Autodesk Inventor part; units mm, degrees
ref_plane "YZ Plane" through (0, 0, 0) normal (1, 0, 0) x (0, 1, 0)
ref_plane "XZ Plane" through (0, 0, 0) normal (0, 1, 0) x (-1, 0, 0)
ref_plane "XY Plane" through (0, 0, 0) normal (0, 0, 1) x (1, 0, 0)
sketch "Sketch1" plane through (0, 0, 0) normal (0, 0, 1) x (1, 0, 0)
  line L0 (0, 0) -> (50.8, 0)
  line L1 (50.8, 0) -> (50.8, 25.4)
  line L2 (50.8, 25.4) -> (0, 25.4)
  line L3 (0, 25.4) -> (0, 0)
  line L4 (3.175, 3.175) -> (47.625, 3.175)
  line L5 (47.625, 3.175) -> (47.625, 22.225)
  line L6 (47.625, 22.225) -> (3.175, 22.225)
  line L7 (3.175, 22.225) -> (3.175, 3.175)
  dimension "d0" = 50.8
  dimension "d1" = 25.4
  dimension "d2" = 44.45
  dimension "d3" = 19.05
  dimension "d4" = 3.175
  dimension "d5" = 3.175
extrude "Extrusion1" add sketch "Sketch1" against normal blind 361.95
sketch "Sketch2" plane through (50.8, 0, 0) normal (1, 0, 0) x (0, 0, -1)
  line L0 (0, 0) -> (0, 25.4)
  line L1 (0, 0) -> (361.95, 0)
  line L2 (361.95, 25.4) -> (361.95, 0)
  line L3 (0, 25.4) -> (361.95, 25.4)
  point P0 (146.05, 12.7)
  point P1 (349.25, 12.7)
  dimension "d8" = 12.7
  dimension "d9" = 12.7
  dimension "d10" = 215.9
  dimension "d11" = 12.7
hole "Hole1" at (50.8, 12.7, -146.05) at (50.8, 12.7, -349.25) direction (-1, 0, 0) diameter 6.35 end through all
sketch "Sketch3" plane through (50.8, 0, 0) normal (1, 0, 0) x (0, 0, -1)
  circle A0 centre (146.05, 12.7) radius 3.175
  circle A1 centre (349.25, 12.7) radius 3.175
  line L0 (0, 0) -> (0, 25.4)
  line L1 (0, 0) -> (361.95, 0)
  line L2 (361.95, 25.4) -> (361.95, 0)
  line L3 (0, 25.4) -> (361.95, 25.4)
  point P0 (12.7, 12.7)
  dimension "d19" = 12.7
  dimension "d20" = 12.7
hole "Hole2" at (50.8, 12.7, -12.7) direction (-1, 0, 0) diameter 6.35 end through all
sketch "Sketch4" plane through (0, 25.4, 0) normal (0, 1, 0) x (1, 0, 0)
  line L0 (50.8, 0) -> (0, 0)
  line L1 (50.8, 0) -> (50.8, 361.95)
  line L2 (0, 361.95) -> (50.8, 361.95)
  line L3 (0, 0) -> (0, 361.95)
  point P0 (25.4, 50.8)
  dimension "d28" = 25.4
  dimension "d29" = 50.8
hole "Hole3" at (25.4, 25.4, -50.8) direction (0, -1, 0) diameter 25.4 end through all
pattern_linear "Rectangular Pattern1" count 8 spacing 38.1 along (0, 0, -1) of "Hole3"
properties part number "2x1 mounting" material "Aluminum 6061"
Work out the finished part from the listing and answer in its coordinate system (mm). Give positions to 0.01 mm unless a question says otherwise; leave off trailing zeros. Loops run counter-clockwise (first coordinate to the right, second up) from the corner with the lowest first, then second, coordinate; pieces in that order, holes last. Notation, with made-up numbers: (50, -32) - (73, -32) arc R18 ccw to (73, -11) - close; hole circle Ø9 at (-8, -28). An arc over 180 degrees is marked (long way). Answer in a Markdown table with one row per item.
(1) Consider L1, parallel to Z at x = 2.55, y = 12.7 (3 decimals); L2, parallel to Y at x = 49.05, z = -12.7 (3 decimals); L3, parallel to X at y = 15, z = -160.5 (3 decimals). Determine where each line is inside the solid, lowest interval first. Write a range as [from, to].
Results list:
| item | result |
|---|---|
| L1 | z = [-361.95, -352.425], [-346.075, -149.225], [-142.875, -15.875], [-9.525, 0] |
| L2 | y = [0, 9.525], [15.875, 25.4] |
| L3 | x = [0, 3.175], [47.625, 50.8] |
(2) Section D-D (z = -165.1) is taken. Give the vertices of the cut face in (x, y) (3 decimals).
Results list:
| item | result |
|---|---|
| outline | (0, 0) - (12.7, 0) - (12.7, 3.175) - (3.175, 3.175) - (3.175, 22.225) - (12.7, 22.225) - (12.7, 25.4) - (0, 25.4) - close; (38.1, 0) - (50.8, 0) - (50.8, 25.4) - (38.1, 25.4) - (38.1, 22.225) - (47.625, 22.225) - (47.625, 3.175) - (38.1, 3.175) - close |
(3) Section B-B (z = -349.25) is taken. Give the vertices of the cut face in (x, y) (3 decimals), and give its area (3 significant figures).
Results list:
| item | result |
|---|---|
| outline | (0, 0) - (50.8, 0) - (50.8, 9.525) - (47.625, 9.525) - (47.625, 3.175) - (3.175, 3.175) - (3.175, 9.525) - (0, 9.525) - close; (0, 15.875) - (3.175, 15.875) - (3.175, 22.225) - (47.625, 22.225) - (47.625, 15.875) - (50.8, 15.875) - (50.8, 25.4) - (0, 25.4) - close |
| area | 403 mm² |
(4) For a pull along X with two mould halves and no side action, classify faces 1 (the face through (1.57, 13.92, -148.98)), 2 (the face through (21.585, 1.565, -305.386)) as pulls with the +X half, pulls with the -X half, needs draft (parallel to the pull), parting line crosses it, or undercut.
Results list:
| item | result |
|---|---|
| face 1 | needs draft |
| face 2 | undercut |
(5) Section A-A (y = 12.7) is taken. State how many separate pieces and enclosed holes the cut face has, and give its area (3 significant figures).
Results list:
| item | result |
|---|---|
| separate pieces | 8 |
| enclosed holes | 0 |
| area | 2,180 mm² |
